Part model, mm, in its own coordinate system. A direction names the side the tool comes from. Give positions to 0.01 mm unless a question says otherwise; leave off trailing zeros. Order: outer loops, then holes, each group sorted by start corner. A loop starts at its lowest first (then second) coordinate and runs counter-clockwise, first axis right, second up.
1. Probe line 1 (X direction, y = 52, z = 73) (3 decimals); line 2 (Y direction, x = -7, z = 24.5) (3 decimals); line 3 (X direction, y = 74.75, z = 50). List the from-to ranges inside material, lowest first.
2. Slice it at B-B on z = 76.5. List the corners of the cut face in (x, y) (3 decimals).
3. Slice it at A-A on y = 60.25. List the corners of the cut face in (x, z) (3 decimals), and give its area (3 significant figures).
4. Which spindle directions (+Z, -Z, +X, -X, +Y, -Y) get a long thin tool onto all of the face, cutting with end or side? Do faces 1 (the flat face through (-34, 73.025, 56)), 2 (the flat face through (-17, 74, 11.753)). Say none if no direction does.
5. Slice it at C-C on x = -31. List the corners of the cut face in (y, z) (3 decimals).
6. Slice it at D-D on z = 64. List the corners of the cut face in (x, y) (3 decimals), and give its area (3 significant figures).
7. Drop flat-ended pins along their axis: pin 1 Ø8 at (y, z) = (64, 52.5) entering from -X (3 decimals); pin 2 Ø6 at (y, z) = (70.5, 49) entering from -X; pin 3 Ø8 at (x, y) = (-53.5, 68) entering from -Z; pin 4 Ø4 at (x, z) = (-27, 77) entering from -Y (3 decimals). Give the stop position or say it passes through.
Autodesk Inventor part; units mm, degrees
ref_plane "Work Plane4" through (-3.175, 0, 101.6) normal (0, -0.7071, 0.7071) x (1, 0, 0)
ref_plane "Work Plane6" through (-63.5, 65.8978, 101.6) normal (0.1262, 0, -0.992) x (0, -1, 0)
ref_plane "Work Plane7" through (0, 50.8, 11.7529) normal (0, -0.7071, -0.7071) x (-1, 0, 0)
sketch "Sketch3" plane through (0, 0, 0) normal (0, 0, 1) x (1, 0, 0)
  line L0 (0, 0) -> (0, 76.2)
  line L1 (0, 76.2) -> (-76.2, 76.2)
  line L2 (-76.2, 73.025) -> (-3.175, 73.025)
  line L3 (-3.175, 73.025) -> (-3.175, 0)
  line L4 (-76.2, 73.025) -> (-76.2, 76.2)
  line L5 (-3.175, 0) -> (0, 0)
  dimension "d8" = 76.2
  dimension "d9" = 76.2
  dimension "d10" = 3.175
extrude "Extrusion2" add sketch "Sketch3" along normal blind 101.6
sketch "Sketch4" plane through (-76.2, 76.2, 0) normal (0, 1, 0) x (1, 0, 0)
  line L0 (24.13, -11.7529) -> (12.7, -101.6)
  line L1 (0, 0) -> (0, -101.6)
  line L2 (24.13, -11.7529) -> (76.2, -11.7529)
  line L3 (76.2, 0) -> (0, 0)
  line L4 (76.2, 0) -> (0, 0)
  line L5 (76.2, 0) -> (76.2, -11.7529)
  line L6 (12.7, -101.6) -> (0, -101.6)
  line L7 (0, 0) -> (0, -101.6)
  line L8 (76.2, 0) -> (76.2, -101.6)
  dimension "d16" = 7.25
  dimension "d17" = 63.5
  dimension "d18" = 52.07
extrude "Extrusion3" cut sketch "Sketch4" against normal blind 76.2
ref_plane "Work Plane4" through (-3.175, 0, 101.6) normal (0, -0.7071, 0.7071) x (1, 0, 0)
ref_plane "Work Plane6" through (-63.5, 65.8978, 101.6) normal (0.1262, 0, -0.992) x (0, -1, 0)
sketch "Sketch6" plane through (0, 0, 101.6) normal (1, 0, 0) x (0, 0, -1)
  line L0 (0, 0) -> (0, 76.2)
  line L1 (0, 50.8) -> (89.8471, 50.8)
  line L2 (89.8471, 0) -> (0, 0)
  line L3 (89.8471, 50.8) -> (89.8471, 0)
  line L4 (89.8471, 0) -> (0, 0)
  line L5 (0, 0) -> (0, 50.8)
  point P0 (101.6, 0)
  dimension "d34" = 50.8
extrude "Extrusion5" cut sketch "Sketch6" against normal blind 25.4
ref_plane "Work Plane7" through (0, 50.8, 11.7529) normal (0, -0.7071, -0.7071) x (-1, 0, 0)
properties part number "BlockForShieldPlacement" material "Aluminum 6061"
Data:
1. line 1: x = -3.175 to 0
1. line 2: y = 73.025 to 76.2
1. line 3: x = -56.94 to 0
2. outline: (-60.307, 73.025) - (-3.175, 73.025) - (-3.175, 50.8) - (0, 50.8) - (0, 76.2) - (-60.307, 76.2) - close
3. outline: (-3.175, 11.753) - (0, 11.753) - (0, 101.6) - (-3.175, 101.6) - close
3. area: 285 mm2
4. face 1: +Z, -Z, -X, -Y
4. face 2: -Z, +X, -X, +Y, -Y
5. outline: (73.025, 11.753) - (76.2, 11.753) - (76.2, 101.6) - (73.025, 101.6) - close
6. outline: (-58.717, 73.025) - (-3.175, 73.025) - (-3.175, 50.8) - (0, 50.8) - (0, 76.2) - (-58.717, 76.2) - close
6. area: 257 mm2
7. pin 1: stops at x = -3.175
7. pin 2: stops at x = -57.01
7. pin 3: passes through
7. pin 4: stops at y = 73.025
